from build123d import *

# Parameters (mm, degrees)
SKETCH1_W           = 70
SKETCH1_H           = 50
BOSS_EXTRUDE1_DEPTH = 1.2
CUT_EXTRUDE1_REACH  = 45.028
SKETCH6_R           = 1.6


with BuildPart() as part:
    # Sketch1 → Boss-Extrude1 (new body)
    with BuildSketch(Plane.XY):
        Rectangle(SKETCH1_W, SKETCH1_H)
    extrude(amount=BOSS_EXTRUDE1_DEPTH)

    # Sketch6 → Cut-Extrude1 (cut, up to next)
    with BuildSketch(Plane.XY.offset(1.2), mode=Mode.PRIVATE) as cut_extrude1_sk1:
        with Locations((-32, -22)):
            Circle(SKETCH6_R)
    cut_extrude1_tool1 = extrude(cut_extrude1_sk1.sketch, amount=-CUT_EXTRUDE1_REACH, mode=Mode.PRIVATE) & part.part
    # Sketch6 → Cut-Extrude1 (cut, up to next)
    with BuildSketch(Plane.XY.offset(1.2), mode=Mode.PRIVATE) as cut_extrude1_sk2:
        with Locations(Location((32, -22, 0), (0, 0, 180))):
            Circle(SKETCH6_R)
    cut_extrude1_tool2 = extrude(cut_extrude1_sk2.sketch, amount=-CUT_EXTRUDE1_REACH, mode=Mode.PRIVATE) & part.part
    # Sketch6 → Cut-Extrude1 (cut, up to next)
    with BuildSketch(Plane.XY.offset(1.2), mode=Mode.PRIVATE) as cut_extrude1_sk3:
        with Locations((32, 22)):
            Circle(SKETCH6_R)
    cut_extrude1_tool3 = extrude(cut_extrude1_sk3.sketch, amount=-CUT_EXTRUDE1_REACH, mode=Mode.PRIVATE) & part.part
    # Sketch6 → Cut-Extrude1 (cut, up to next)
    with BuildSketch(Plane.XY.offset(1.2), mode=Mode.PRIVATE) as cut_extrude1_sk4:
        with Locations(Location((-32, 22, 0), (0, 0, 180))):
            Circle(SKETCH6_R)
    cut_extrude1_tool4 = extrude(cut_extrude1_sk4.sketch, amount=-CUT_EXTRUDE1_REACH, mode=Mode.PRIVATE) & part.part
    add(cut_extrude1_tool1.solids().sort_by_distance((-32, -22, 1.2))[0], mode=Mode.SUBTRACT)
    add(cut_extrude1_tool2.solids().sort_by_distance((32, -22, 1.2))[0], mode=Mode.SUBTRACT)
    add(cut_extrude1_tool3.solids().sort_by_distance((32, 22, 1.2))[0], mode=Mode.SUBTRACT)
    add(cut_extrude1_tool4.solids().sort_by_distance((-32, 22, 1.2))[0], mode=Mode.SUBTRACT)


solid = part.part
Could you check a few things on this model? Use its own coordinates, in mm. Give positions to 0.01 mm unless a question says otherwise; leave off trailing zeros. Order: outer loops, then holes, each group sorted by start corner. A loop starts at its lowest first (then second) coordinate and runs counter-clockwise, first axis right, second up.
1. Suppose I cut it at B-B (y = 22). Write out the boundary of the cut face in (x, z), plus the area to 3 significant figures.
Answers below:
outline: (-35, 0) - (-33.6, 0) - (-33.6, 1.2) - (-35, 1.2) - close; (-30.4, 0) - (30.4, 0) - (30.4, 1.2) - (-30.4, 1.2) - close; (33.6, 0) - (35, 0) - (35, 1.2) - (33.6, 1.2) - close
area: 76.3 mm2
2. Suppose I cut it at A-A (x = 32). Write out the boundary of the cut face in (y, z).
Answers below:
outline: (-25, 0) - (-23.6, 0) - (-23.6, 1.2) - (-25, 1.2) - close; (-20.4, 0) - (20.4, 0) - (20.4, 1.2) - (-20.4, 1.2) - close; (23.6, 0) - (25, 0) - (25, 1.2) - (23.6, 1.2) - close
3. I need wall thicknesses on L1, parallel to Y at x = -32, z = 0.35; L2, parallel to Y at x = -31, z = 0.65. Which ranges of each line are inside material? Lowest first, please.
Answers below:
L1: y = -25 to -23.6, -20.4 to 20.4, 23.6 to 25
L2: y = -25 to -23.25, -20.75 to 20.75, 23.25 to 25
4. Thinking about a two-plate mould opening in Y: for faces 1 (the cylindrical face through (33.18, -23.08, 0.61)), 2 (the cylindrical face through (-30.82, 20.92, 0.61)), 3 (the flat face through (0, 0, 0)), which applies, +Y half, -Y half, draft (parallel to the pull), parting line (faces both ways), or undercut?
Answers below:
face 1: undercut
face 2: undercut
face 3: draft
